from build123d import *

# Parameters (mm, degrees)
SKETCH1_R           = 31.5
BOSS_EXTRUDE1_DEPTH = 25
SHELL1_T            = -5
SKETCH2_R           = 5
BOSS_EXTRUDE3_DEPTH = 20


with BuildPart() as part:
    # Sketch1 → Boss-Extrude1 (new, symmetric)
    with BuildSketch(Plane(origin=(0, 0, 0), x_dir=(0, 0, -1), z_dir=(1, 0, 0))):
        Circle(SKETCH1_R)
    extrude(amount=BOSS_EXTRUDE1_DEPTH, both=True)

    # Shell1
    shell1_openings = [part.faces().sort_by_distance(p)[0] for p in [
        (-25, 0, 0),
    ]]
    offset(amount=SHELL1_T, openings=shell1_openings, kind=Kind.INTERSECTION)

    # Sketch2 → Boss-Extrude3 (add)
    with BuildSketch(Plane(origin=(25, 0, 0), x_dir=(0, 0, -1), z_dir=(1, 0, 0))):
        Circle(SKETCH2_R)
    extrude(amount=BOSS_EXTRUDE3_DEPTH)


solid = part.part
Can you work these out from the model? Positions are in its coordinate system, mm. Coordinates: 2 decimals unless noted, no trailing zeros. Write each loop counter-clockwise with the first axis right and the second up, starting at its lowest first coordinate (ties: lowest second). Pieces come first, ordered by that corner, then holes. Notation, with made-up numbers: M -26,30 L 29,30 A3 ccw 29,35 Z; hole C 71,36 d2. An arc over 180 degrees is marked long. Use one line per item in the form item = value.
Q1. I need wall thicknesses on line 1 along Y through (x, z) = (-2, 0); line 2 along X through (y, z) = (9, -23); line 3 along X through (y, z) = (-29, -2). Which ranges of each line are inside material? Lowest first, please. Write a range as from..to.
Model answer:
line_1 = -31.5..-26.5, 26.5..31.5
line_2 = 20..25
line_3 = -25..25
Q2. If we section it at D-D (x = 37): Write out the boundary of the cut face in (y, z), then the cut area to 3 significant figures.
Model answer:
outline = C 0,0 d10
area = 78.5 mm^2
Q3. If we section it at C-C (x = 6): Write out the boundary of the cut face in (y, z), then the cut area to 3 significant figures.
Model answer:
outline = C 0,0 d63; hole C 0,0 d53
area = 911 mm^2
Q4. If we section it at B-B (z = 12.5): Write out the boundary of the cut face in (x, y).
Model answer:
outline = M -25,-28.91 L 25,-28.91 L 25,28.91 L -25,28.91 L -25,23.37 L 20,23.37 L 20,-23.37 L -25,-23.37 Z
Q5. For P1, Ø1.5, axis at y = 8.5, z = -11, coming from the -X side; P2, Ø8, axis at x = 7.5, z = 2.5, coming from the +Y side; P3, Ø4, axis at x = 21.5, y = 4, coming from the -Z side, each with a flat end and sliding along its axis, tell me the tip position at first contact or that it passes through.
Model answer:
P1 = 20
P2 = 31.5
P3 = -31.44
Q6. If we section it at A-A (y = 0): Write out the boundary of the cut face in (x, z), then the cut area to 3 significant figures.
Model answer:
outline = M -25,-31.5 L 25,-31.5 L 25,-5 L 45,-5 L 45,5 L 25,5 L 25,31.5 L -25,31.5 L -25,26.5 L 20,26.5 L 20,-26.5 L -25,-26.5 Z
area = 965 mm^2
Q7. We'd pull the mould along Z, two halves only. Please class faces 1 (the flat face through (25, 0, -7)), 2 (the cylindrical face through (34.86, -4.88, 1.08)), 3 (the cylindrical face through (-2.185, 22.345, -14.246)), 4 (the flat face through (20, 0, 0)): +Z half, -Z half, draft (parallel to the pull), parting line (faces both ways), or undercut.
Model answer:
face_1 = draft
face_2 = parting line
face_3 = undercut
face_4 = undercut
